from build123d import *
from build123d.topology import SkipClean

# Parameters (mm, degrees)
SKETCH1_R           = 10
BOSS_EXTRUDE1_DEPTH = 2.5
BOSS_EXTRUDE2_DEPTH = 25
SKETCH5_R           = 1.587
BOSS_EXTRUDE3_DEPTH = 10
CIRPATTERN2_COUNT   = 4


with BuildPart() as part:
    # Sketch1 → Boss-Extrude1 (new body)
    with BuildSketch(Plane(origin=(0, 0, 0), x_dir=(1, 0, 0), z_dir=(0, 1, 0))):
        with Locations(Location((0, 0, 0), (0, 0, 270))):
            Circle(SKETCH1_R)
    extrude(amount=BOSS_EXTRUDE1_DEPTH)

    # Sketch3 → Boss-Extrude2 (add)
    with BuildSketch(Plane(origin=(0, 2.5, 0), x_dir=(1, 0, 0), z_dir=(0, 1, 0))):
        with BuildLine():
            Line((-7.660254038, 5), (-8.660254038, 5))
            ThreePointArc((-8.660254038, 5), (-10, 0), (-8.660254038, -5))
            Line((-8.660254038, -5), (-7.660254038, -5))
            Line((-7.660254038, -5), (-7.660254038, 5))
        make_face()
        with BuildLine():
            Line((-5, -7.660254038), (-5, -8.660254038))
            ThreePointArc((-5, -8.660254038), (0, -10), (5, -8.660254038))
            Line((5, -8.660254038), (5, -7.660254038))
            Line((5, -7.660254038), (-5, -7.660254038))
        make_face()
        with BuildLine():
            ThreePointArc((10, 0), (9.659258263, 2.588190451), (8.660254038, 5))
            Line((8.660254038, 5), (7.660254038, 5))
            Line((7.660254038, 5), (7.660254038, -5))
            Line((7.660254038, -5), (8.660254038, -5))
            ThreePointArc((8.660254038, -5), (9.659258263, -2.588190451), (10, 0))
        make_face()
        with BuildLine():
            ThreePointArc((5, 8.660254038), (0, 10), (-5, 8.660254038))
            Line((-5, 8.660254038), (-5, 7.660254038))
            Line((-5, 7.660254038), (5, 7.660254038))
            Line((5, 7.660254038), (5, 8.660254038))
        make_face()
    extrude(amount=BOSS_EXTRUDE2_DEPTH)

    # Sketch5 → Boss-Extrude3 (add)
    with BuildSketch(Plane(origin=(0, 0, 0), x_dir=(-1, 0, 0), z_dir=(0, -1, 0))):
        with Locations(Location((0, 0, 0), (0, 0, 90))):
            Circle(SKETCH5_R)
    extrude(amount=BOSS_EXTRUDE3_DEPTH)

    # Sketch7 → Cut-Revolve1 (revolve, cut)
    with BuildSketch(Plane(origin=(0, 15, 0), x_dir=(1, 0, 0), z_dir=(0, 1, 0))):
        Polygon((0, 7.660254038), (1.75, 7.660254038), (1.75, 8.660254038), (3.55, 8.660254038), (3.55, 10.3184344), (0, 10.3184344), align=None)
    cut_revolve1 = revolve(axis=Axis((0, 15, 0), (0, 0, -1)), mode=Mode.SUBTRACT)

    # CirPattern2: Cut-Revolve1 ×4 about axis
    with SkipClean():  # the faces are left unmerged after this step: merging them gives an invalid solid
        cirpattern2_axis = Axis((0, 0, 0), (0, 1, 0))
        for i in range(1, CIRPATTERN2_COUNT):
            add(cut_revolve1.rotate(cirpattern2_axis, i * 360 / CIRPATTERN2_COUNT), mode=Mode.SUBTRACT)


solid = part.part
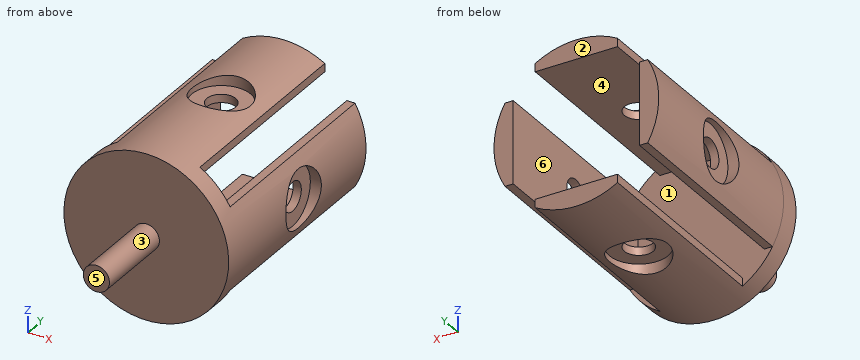
Can you work these out from the model? Positions are in its coordinate system, mm. Face numbers are marked on the shaded views. A direction names the side the tool comes from. Coordinates: 2 decimals unless noted, no trailing zeros. Write each loop counter-clockwise with the first axis right and the second up, starting at its lowest first coordinate (ties: lowest second). Pieces come first, ordered by that corner, then holes. Notation, with made-up numbers: M 23.5,-8.5 L 47.5,-8.5 A17 ccw 47.5,20.5 Z; hole C 22.25,74.25 d9. An arc over 180 degrees is marked long. Use one line per item in the form item = value.
Q1. For the marked faces 4, 5 and 6, which set-ups out of +Z, -Z, +X, -X, +Y, -Y let a thin tool reach every point of the face, with its end or its side?
Model answer:
face_4 = +X, -X, +Y
face_5 = +Z, -Z, +X, -X, -Y
face_6 = +Z, -Z, +Y
Q2. If we section it at D-D (x = 6): Write out the boundary of the cut face in (y, z).
Model answer:
outline = M 0,-8 L 2.5,-8 L 2.5,8 L 0,8 Z
Q3. For P1, Ø3, axis at x = 0, y = 15, coming from the +Z side; P2, Ø0.5, axis at x = -8, y = 9, coming from the -Z side; P3, Ø5.5, axis at x = 0, y = 14.5, coming from the +Z side; P4, Ø1, axis at x = -5, z = -0.5, coming from the +Y side, each with a flat end and sliding along its axis, tell me the tip position at first contact or that it passes through.
Model answer:
P1 = through
P2 = -5
P3 = 8.66
P4 = 2.5
Q4. If we section it at C-C (z = 0): Write out the boundary of the cut face in (x, y).
Model answer:
outline = M -10,0 L -1.59,0 L -1.59,-10 L 1.59,-10 L 1.59,0 L 10,0 L 10,11.45 L 8.66,11.45 L 8.66,13.25 L 7.66,13.25 L 7.66,2.5 L -7.66,2.5 L -7.66,13.25 L -8.66,13.25 L -8.66,11.45 L -10,11.45 Z; M -10,18.55 L -8.66,18.55 L -8.66,16.75 L -7.66,16.75 L -7.66,27.5 L -10,27.5 Z; M 7.66,16.75 L 8.66,16.75 L 8.66,18.55 L 10,18.55 L 10,27.5 L 7.66,27.5 Z
Q5. We'd pull the mould along Z, two halves only. Please class the marked faces 1, 2 and 3: +Z half, -Z half, draft (parallel to the pull), parting line (faces both ways), or undercut.
Model answer:
face_1 = undercut
face_2 = draft
face_3 = parting line
Q6. I need wall thicknesses on line 1 along Y through (x, z) = (0, 9.6); line 2 along Z through (x, y) = (-7.85, 15); line 3 along Y through (x, z) = (7.95, 0). Which ranges of each line are inside material? Lowest first, please. Write a range as from..to.
Model answer:
line_1 = 0..11.45, 18.55..27.5
line_2 = -5..-1.75, 1.75..5
line_3 = 0..13.25, 16.75..27.5
Q7. If we section it at B-B (y = 5): Write out the boundary of the cut face in (x, z).
Model answer:
outline = M -8.66,-5 L -7.66,-5 L -7.66,5 L -8.66,5 A10 ccw Z; M -5,-8.66 A10 ccw 5,-8.66 L 5,-7.66 L -5,-7.66 Z; M -5,7.66 L 5,7.66 L 5,8.66 A10 ccw -5,8.66 Z; M 7.66,-5 L 8.66,-5 A10 ccw 8.66,5 L 7.66,5 Z
Q8. If we section it at A-A (x = 0): Write out the boundary of the cut face in (y, z), then the cut area to 3 significant figures.
Model answer:
outline = M -10,-1.59 L 0,-1.59 L 0,-10 L 11.45,-10 L 11.45,-8.66 L 13.25,-8.66 L 13.25,-7.66 L 2.5,-7.66 L 2.5,7.66 L 13.25,7.66 L 13.25,8.66 L 11.45,8.66 L 11.45,10 L 0,10 L 0,1.59 L -10,1.59 Z; M 16.75,-8.66 L 18.55,-8.66 L 18.55,-10 L 27.5,-10 L 27.5,-7.66 L 16.75,-7.66 Z; M 16.75,7.66 L 27.5,7.66 L 27.5,10 L 18.55,10 L 18.55,8.66 L 16.75,8.66 Z
area = 173 mm^2
